Autodesk Inventor part; units mm, degrees
ref_plane "YZ Plane" through (0, 0, 0) normal (1, 0, 0) x (0, 1, 0)
ref_plane "XZ Plane" through (0, 0, 0) normal (0, 1, 0) x (-1, 0, 0)
ref_plane "XY Plane" through (0, 0, 0) normal (0, 0, 1) x (1, 0, 0)
sketch "Sketch6" plane through (0, 1.5, 0) normal (0, 1, 0) x (1, 0, 0)
  line L0 (-131, 222) -> (-131, -12)
  line L1 (-131, 152) -> (-134, 152)
  line L2 (-134, 152) -> (-134, 92)
  line L3 (-134, 92) -> (-131, 92)
  line L4 (-131, 92) -> (-131, 152)
  line L5 (-87, 222) -> (-131, 222)
  line L6 (-109, 222) -> (-109, 171)
  line L7 (-124.04, 171) -> (-93.96, 171)
  line L8 (-87, 152) -> (-84, 152)
  line L9 (-84, 152) -> (-84, 92)
  line L10 (-84, 92) -> (-87, 92)
  line L11 (-87, 92) -> (-87, 152)
  point P0 (0, 0)
  point P1 (-134, 122)
  point P2 (-84, 122)
  dimension "d38" = 3
  dimension "d39" = 60
  dimension "d40" = 100
sketch "Sketch1" plane through (0, 0, 0) normal (0, 1, 0) x (-1, 0, 0)
  line L0 (-241, 22) -> (241, 22)
  line L1 (241, 22) -> (241, -22)
  line L2 (241, -22) -> (-241, -22)
  line L3 (-241, -22) -> (-241, 22)
  line L4 (-241, 22) -> (241, -22) construction
  line L5 (241, 22) -> (-241, -22) construction
  line L6 (50, -22) -> (-50, -22)
  line L7 (-50, -22) -> (-50, -25.5)
  line L8 (-50, -25.5) -> (50, -25.5)
  line L9 (50, -25.5) -> (50, -22)
  line L10 (50, -22) -> (-50, -25.5) construction
  line L11 (-50, -22) -> (50, -25.5) construction
  line L12 (241, 0) -> (-241, 0)
  line L13 (50, 22) -> (-50, 22)
  line L14 (-50, 22) -> (-50, 25.5)
  line L15 (-50, 25.5) -> (50, 25.5)
  line L16 (50, 25.5) -> (50, 22)
  line L17 (50, 22) -> (-50, 25.5) construction
  line L18 (-50, 22) -> (50, 25.5) construction
  line L19 (121, 15) -> (115.8, 15)
  line L20 (115.8, 15) -> (115.8, -15)
  line L21 (115.8, -15) -> (121, -15)
  line L22 (121, -15) -> (121, 15)
  line L23 (121, 15) -> (115.8, -15) construction
  line L24 (115.8, 15) -> (121, -15) construction
  circle A0 centre (0, -19) radius 1.6
  circle A1 centre (0, 19) radius 1.6
  line L25 (131, -22) -> (131, 22)
  point P0 (0, 0)
  point P1 (0, -23.75)
  point P2 (0, -22)
  point P3 (0, 23.75)
  point P4 (0, 22)
  point P5 (50, -22)
  point P6 (50, 22)
  point P7 (-50, 22)
  point P8 (-50, -22)
  point P9 (118.4, 0)
  point P10 (0, 0)
  dimension "d0" = 482
  dimension "d1" = 44
  dimension "d2" = 100
  dimension "d3" = 3.5
  dimension "d5" = 5.2
  dimension "d6" = 30
  dimension "d8" = 3.2
  dimension "d9" = 38
  dimension "d23" = 10
  dimension "d24" = 110
extrude "Plate1" add sketch "Sketch1" along normal mid plane 3 contours L0 L25 L12 L22 L19 L20 L3 | L14 L15 L16 L0 | L12 L20 L21 L22 L25 L2 L3 | L20 L19 L22 L12 | L12 L22 L21 L20 | L2 L9 L8 L7
sketch "Sketch2" plane through (0, 1.5, 0) normal (0, 1, 0) x (1, 0, 0)
  line L0 (0, -3.5) -> (0, 3.5) construction
  line L1 (5, -3.5) -> (5, 3.5)
  line L2 (-5, 3.5) -> (-5, -3.5)
  arc A0 (-5, -3.5) -> (5, -3.5) centre (0, -3.5) ccw
  arc A1 (5, 3.5) -> (-5, 3.5) centre (0, 3.5) ccw
  line L3 (-50, -25.5) -> (50, -25.5)
  line L4 (25, -25.5) -> (25, 25.5)
  line L5 (50, 25.5) -> (-50, 25.5)
  circle A2 centre (0, -19) radius 1.6
  line L6 (50, -3.5) -> (50, 3.5) construction
  line L7 (45, -3.5) -> (45, 3.5)
  line L8 (55, 3.5) -> (55, -3.5)
  arc A3 (45, -3.5) -> (55, -3.5) centre (50, -3.5) ccw
  arc A4 (55, 3.5) -> (45, 3.5) centre (50, 3.5) ccw
  point P0 (0, 0)
  point P1 (0, 8.5)
  point P2 (0, -8.5)
  point P3 (50, 0)
  point P4 (50, 8.5)
  point P5 (50, -8.5)
  dimension "d10" = 17
  dimension "d11" = 5
  dimension "d12" = 25
extrude "Cut1" cut sketch "Sketch2" against normal blind 3 contours A0 L2 A1 L1 | L7 A4 L8 A3
sketch "Sketch3" plane through (0, 1.5, 0) normal (0, 1, 0) x (1, 0, 0)
  line L0 (-50, -25.5) -> (50, -25.5)
  line L1 (0, -25.5) -> (0, 25.5)
  line L2 (50, 25.5) -> (-50, 25.5)
  line L3 (-241, 0) -> (241, 0)
  line L4 (241, -22) -> (241, 22)
  line L5 (50, 22) -> (-50, 22)
  line L6 (191, 22) -> (111, 22)
  line L7 (111, 22) -> (111, 26)
  line L8 (111, 26) -> (191, 26)
  line L9 (191, 26) -> (191, 22)
  line L10 (191, -26) -> (191, -22)
  line L11 (191, -22) -> (111, -22)
  line L12 (111, -22) -> (111, -26)
  line L13 (111, -26) -> (191, -26)
  point P0 (0, 0)
  point P1 (151, 22)
  point P2 (151, -22)
sheet face with bend "Face2" sketch "Sketch3" thickness 3 toward (0, -1, 0) bend radius 3
bend "Bend1"
sketch "Sketch4" plane through (0, 1.5, 0) normal (0, 1, 0) x (1, 0, 0)
  line L0 (-50, 22) -> (-131, 22)
  line L1 (-131, 22) -> (-87, 22)
  line L2 (-87, 22) -> (-87, 222)
  line L3 (-87, 222) -> (-131, 222)
  line L4 (-131, 222) -> (-131, 22)
  point P0 (0, 0)
  dimension "d25" = 44
  dimension "d26" = 200
sheet face with bend "Face3" sketch "Sketch4" thickness 3 toward (0, -1, 0) bend radius 3
bend "Bend2"
fillet "Corner Round1" radius 10 2 edges at (-87, 0, -22) (-131, 0, 22)
sketch "Sketch5" plane through (0, 1.5, 0) normal (0, 1, 0) x (1, 0, 0)
  line L0 (-124.04, 181) -> (-93.96, 181)
  line L1 (-93.96, 181) -> (-93.96, 171)
  line L2 (-93.96, 171) -> (-124.04, 171)
  line L3 (-124.04, 171) -> (-124.04, 181)
  line L4 (-87, 222) -> (-131, 222)
  point P0 (0, 0)
  point P1 (-109, 222)
  point P2 (-109, 181)
  dimension "d33" = 41
  dimension "d34" = 10
  dimension "d35" = 30.08
extrude "Cut2" cut sketch "Sketch5" against normal blind 3
sheet face with bend "Face4" sketch "Sketch6" thickness 3 toward (0, -1, 0) bend radius 3
bend "Bend3"
equation "\"d13\" = Thickness"
equation "\"d36\" = Thickness"
equation "\"d4\" = Thickness"
equation "\"d18\" = BendRadius"
equation "\"d19\" = BendReliefWidth"
equation "\"d21\" = MinimumRemnant"
equation "\"d20\" = BendReliefDepth"
equation "\"d22\" = TransitionRadius"
equation "\"d27\" = BendRadius"
equation "\"d28\" = BendReliefWidth"
equation "\"d30\" = MinimumRemnant"
equation "\"d29\" = BendReliefDepth"
equation "\"d31\" = TransitionRadius"
equation "\"d41\" = BendRadius"
equation "\"d42\" = BendReliefWidth"
equation "\"d44\" = MinimumRemnant"
equation "\"d43\" = BendReliefDepth"
equation "\"d45\" = TransitionRadius"
equation "\"BendRadius\" = Thickness"
equation "\"BendReliefWidth\" = Thickness"
equation "\"BendReliefDepth\" = 0.5 * Thickness"
equation "\"CornerReliefSize\" = 4 * Thickness"
equation "\"MinimumRemnant\" = 2 * Thickness"
equation "\"TransitionRadius\" = BendRadius"
equation "\"JacobiRadiusSize\" = BendRadius"
equation "\"GapSize\" = Thickness"
properties part number "Path"
Source: CAD feature listing. Evaluate the final solid. Frame: model axes, mm. Give positions to 0.01 mm unless a question says otherwise; leave off trailing zeros. Order: outer loops, then holes, each group sorted by start corner. A loop starts at its lowest first (then second) coordinate and runs counter-clockwise, first axis right, second up. Notation, with made-up numbers: (23, -15) -> (71, -15) arc R4 ccw to (71, -8) -> close; hole circle Ø4 at (89, 5.25). An arc over 180 degrees is marked (long way). Use a Markdown table: item, result.
Q1. Section A-A (x = 30). Return the cut outline in (y, z).
A:
| item | result |
|---|---|
| outline | (-1.5, -25.5) -> (1.5, -25.5) -> (1.5, 25.5) -> (-1.5, 25.5) -> close |
Q2. Material intervals for line 1 (Z direction, x = -107, y = -0.95); line 2 (Z direction, x = 0, y = 0.95); line 3 (X direction, y = 0.1, z = -5.5), sorted ascending. Write a range as [from, to].
A:
| item | result |
|---|---|
| line 1 | [-222, -181], [-171, 22] |
| line 2 | [-25.5, -20.6], [-17.4, -8.5], [8.5, 17.4], [20.6, 25.5] |
| line 3 | [-131, -4.58], [4.58, 45.42], [54.58, 241] |
Q3. Section B-B (z = -199.5). Return the cut outline in (x, y).
A:
| item | result |
|---|---|
| outline | (-131, -1.5) -> (-87, -1.5) -> (-87, 1.5) -> (-131, 1.5) -> close |
Q4. Section C-C (y = -0.2). State how many separate pieces and enclosed holes the cut face has, and give its area (3 significant figures).
A:
| item | result |
|---|---|
| separate pieces | 1 |
| enclosed holes | 5 |
| area | 26,300 mm^2 |
Q5. Pull-direction query (X, two-part tool) for faces 1 (the face through (-128.15, 0.02, 18.99)), 2 (the face through (-83.99, -0.02, -24.85)), 3 (the face through (-3, 1.5, -25)); classes: +X half, -X half, draft (parallel to the pull), parting line (faces both ways), or undercut.
A:
| item | result |
|---|---|
| face 1 | -X half |
| face 2 | undercut |
| face 3 | draft |
Q6. First-contact query: P1, Ø1.5, axis at y = -0.5, z = -200, coming from the -X side; P2, Ø1.5, axis at y = -0.5, z = -24.5, coming from the +X side; P3, Ø1.5, axis at y = 1, z = -196.5, coming from the +X side. Flat tips, straight axial feed; report the tip coordinate or a pass-through.
A:
| item | result |
|---|---|
| P1 | x = -131 |
| P2 | x = 191 |
| P3 | x = -87 |
